The model under review builds one solid part; all positions refer to its coordinate system, in mm. A direction names the side the tool comes from. Round coordinates to 2 decimals unless told otherwise and drop trailing zeros. Loops run counter-clockwise (first coordinate to the right, second up) from the corner with the lowest first, then second, coordinate; pieces in that order, holes last. Notation, with made-up numbers: (-7.75, 40) -> (18.25, 40) arc R29 ccw to (18.25, 74) -> close; hole circle Ø10 at (74, 13). An arc over 180 degrees is marked (long way). Use CSV: the item, a comma, the result in double quotes. Start each with the question number.
```python
from build123d import *

# Parameters (mm, degrees)
SKETCH2_W           = 19.05
SKETCH2_H           = 38.1
SKETCH2_W_2         = 15.875
SKETCH2_H_2         = 34.925
EXTRUDE_THIN1_DEPTH = 456.184
SKETCH3_R           = 14.2875
CUT_EXTRUDE1_DEPTH  = 20.05


with BuildPart() as part:
    # Sketch2 → Extrude-Thin1 (new body)
    with BuildSketch(Plane(origin=(0, 0, 0), x_dir=(1, 0, 0), z_dir=(0, 1, 0))):
        with Locations((9.525, 19.05)):
            Rectangle(SKETCH2_W, SKETCH2_H)
        with Locations((9.525, 19.05)):
            Rectangle(SKETCH2_W_2, SKETCH2_H_2, mode=Mode.SUBTRACT)
    extrude(amount=EXTRUDE_THIN1_DEPTH)

    # Sketch3 → Cut-Extrude1 (cut, through all)
    with BuildSketch(Plane.ZY):
        with Locations((-19.05, 19.05)):
            Circle(SKETCH3_R)
        with BuildLine():
            ThreePointArc((-19.05, 0), (-32.520384182, 5.579615818), (-38.1, 19.05))
            Line((-38.1, 19.05), (-38.1, 0))
            Line((-38.1, 0), (-19.05, 0))
        make_face()
        with BuildLine():
            ThreePointArc((0, 19.05), (-5.579615818, 5.579615818), (-19.05, 0))
            Line((-19.05, 0), (0, 0))
            Line((0, 0), (0, 19.05))
        make_face()
        with Locations((-19.05, 437.134)):
            Circle(SKETCH3_R)
        with BuildLine():
            Line((-38.1, 456.184), (-38.1, 437.134))
            ThreePointArc((-38.1, 437.134), (-32.520384182, 450.604384182), (-19.05, 456.184))
            Line((-19.05, 456.184), (-38.1, 456.184))
        make_face()
        with BuildLine():
            Line((0, 456.184), (-19.05, 456.184))
            ThreePointArc((-19.05, 456.184), (-5.579615818, 450.604384182), (0, 437.134))
            Line((0, 437.134), (0, 456.184))
        make_face()
    extrude(amount=-CUT_EXTRUDE1_DEPTH, mode=Mode.SUBTRACT)


solid = part.part
```
1. Take a section at B-B, the plane x = 10.25. Give the boundary of the cut face in (y, z), then the cut area to 3 significant figures.
2. The part is to be moulded in two halves that separate along Z. For faces 1 (the face through (9, 225, -38.1)), 2 (the face through (19.05, 225, -19)), 3 (the face through (18.25, 13.58, -5.85)), say which applies: pulls with the +Z half, pulls with the -Z half, needs draft (parallel to the pull), parting line crosses it, or undercut.
3. For faces 4 (the face through (17.462, 225, -19)), 5 (the face through (0, 225, -19)), list the 3-axis set-ups (+Z, -Z, +X, -X, +Y, -Y) from which the entire face can be reached by the end or side of a thin tool; tool diameter is ignored.
4. Take a section at C-C, the plane z = -29.5. Give the boundary of the cut face in (x, y), then the cut area to 3 significant figures.
5. For line 1 along Y through (x, z) = (17.9, -19.05); line 2 along X through (y, z) = (269, -20); line 3 along Z through (x, y) = (9.75, 353), list the stretches that pass through material, from the lowest coordinate up. Write a range as from..to.
6. Take a section at A-A, the plane y = 130.5. Give the boundary of the cut face in (x, z), then the cut area to 3 significant figures.
Results:
1,outline,"(11.44, -36.51) arc R19.05 ccw to (19.05, -38.1) -> (437.13, -38.1) arc R19.05 ccw to (444.75, -36.51) -> close; (11.44, -1.59) -> (444.75, -1.59) arc R19.05 ccw to (437.13, 0) -> (19.05, 0) arc R19.05 ccw to start"
1,area,"1,360 mm²"
2,face 1,"pulls with the -Z half"
2,face 2,"needs draft"
2,face 3,"undercut"
3,face 4,"+Y, -Y"
3,face 5,"+Z, -Z, -X, +Y, -Y"
4,outline,"(0, 3.12) -> (1.59, 3.12) -> (1.59, 9.31) -> (0, 9.31) -> close; (0, 28.79) -> (1.59, 28.79) -> (1.59, 427.39) -> (0, 427.39) -> close; (0, 446.88) -> (1.59, 446.88) -> (1.59, 453.06) -> (0, 453.06) -> close; (17.46, 3.12) -> (19.05, 3.12) -> (19.05, 9.31) -> (17.46, 9.31) -> close; (17.46, 28.79) -> (19.05, 28.79) -> (19.05, 427.39) -> (17.46, 427.39) -> close; (17.46, 446.88) -> (19.05, 446.88) -> (19.05, 453.06) -> (17.46, 453.06) -> close"
4,area,"1,300 mm²"
5,line 1,"0..4.76, 33.34..422.85, 451.42..456.18"
5,line 2,"0..1.59, 17.46..19.05"
5,line 3,"-38.1..-36.51, -1.59..0"
6,outline,"(0, -38.1) -> (19.05, -38.1) -> (19.05, 0) -> (0, 0) -> close; hole (1.59, -36.51) -> (17.46, -36.51) -> (17.46, -1.59) -> (1.59, -1.59) -> close"
6,area,"171 mm²"
